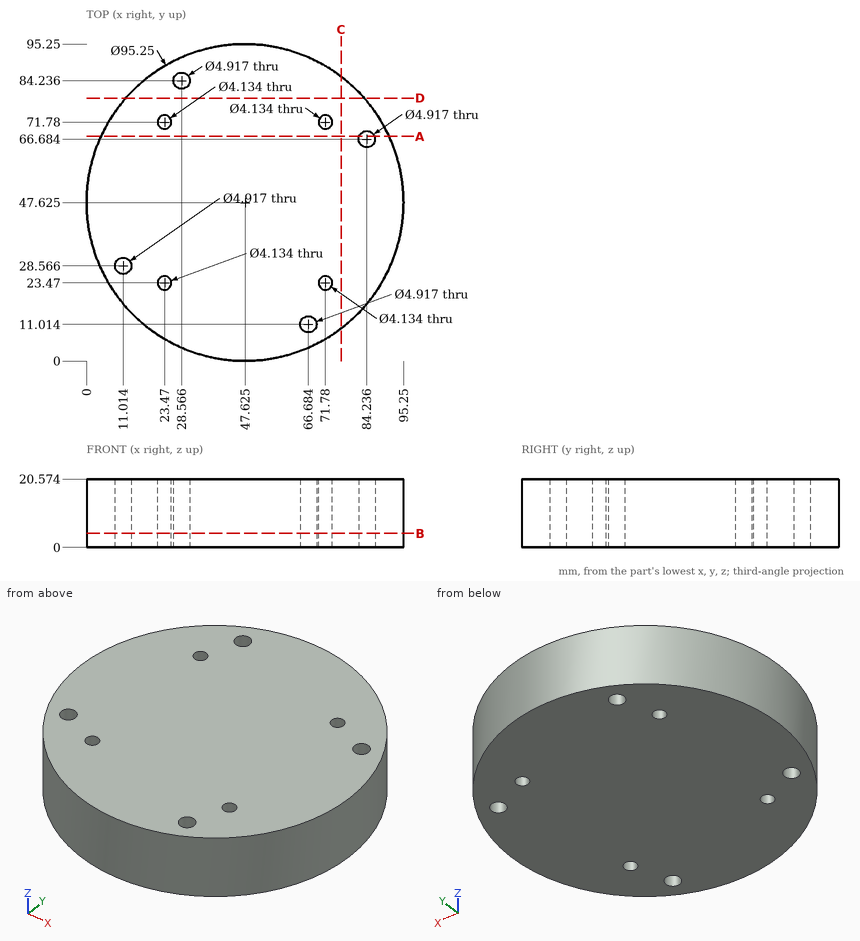
Design review of the part shown in the three views and the two pictorial views. Dimensions are in mm from the part's minimum x, y and z. Give positions to 0.01 mm unless a question says otherwise; leave off trailing zeros. Write each loop counter-clockwise with the first axis right and the second up, starting at its lowest first coordinate (ties: lowest second). Pieces come first, ordered by that corner, then holes. Notation, with made-up numbers: M 0,-29.5 L 59,-29.5 A23 ccw 59,-19.5 Z; hole C 83,12.25 d11. An arc over 180 degrees is marked long. One line per question, with ' | ' between items. Start each with the question number.
Item 1: We need section A-A on y = 67.5. Write out the cut boundary in (x, z) (1 decimal), plus the area to 3 significant figures.
Item 2: Wall thickness on line 1 (Y direction, x = 64.5, z = 5) (1 decimal); line 2 (X direction, y = 67.5, z = 17.5) (1 decimal); line 3 (Y direction, x = 86.5, z = 3.5) (1 decimal): over which ranges is each line inside the solid? List them lowest first. Write a range as from..to.
Item 3: We need section B-B on z = 4.25. Give the number of separate pieces and of enclosed holes in the cut face, plus the area to 3 significant figures.
Item 4: For pin 1 (3 mm diameter, centred on x = 11.01, y = 28.57, fed in from -Z); pin 2 (4 mm diameter, centred on x = 33.5, y = 64, fed in from -Z); pin 3 (8 mm diameter, centred on x = 40, z = 12.5, fed in from -Y); pin 4 (4 mm diameter, centred on y = 12.5, z = 11.5, fed in from -X), all flat-tipped, find the tip position at first contact; note any pin that passes through.
Item 5: We need section C-C on x = 76.5. Write out the cut boundary in (y, z).
Item 6: We need section D-D on y = 79. Write out the cut boundary in (x, z) (1 decimal).
Results found:
1) outline: M 4.3,0 L 81.9,0 L 81.9,20.6 L 4.3,20.6 Z; M 86.6,0 L 90.9,0 L 90.9,20.6 L 86.6,20.6 Z | area: 1,690 mm2
2) line 1: y = 3.1..9.9, 12.1..92.2 | line 2: x = 4.3..81.9, 86.6..90.9 | line 3: y = 20.1..65.7, 67.6..75.1
3) separate pieces: 1 | enclosed holes: 8 | area: 7,000 mm2
4) pin 1: passes through | pin 2: stops at z = 0 | pin 3: stops at y = 0.14 | pin 4: stops at x = 13.41
5) outline: M 9.75,0 L 85.5,0 L 85.5,20.57 L 9.75,20.57 Z
6) outline: M 11.8,0 L 83.5,0 L 83.5,20.6 L 11.8,20.6 Z
